For this review, take the finished solid that the model builds, in its own axes (mm). Coordinates: 2 decimals unless noted, no trailing zeros. Write each loop counter-clockwise with the first axis right and the second up, starting at its lowest first coordinate (ties: lowest second). Pieces come first, ordered by that corner, then holes.
1) To check wall thickness, follow line 1 along Y through (x, z) = (-34, 2.15); line 2 along Y through (x, z) = (-18.5, 2.45) (3 decimals); line 3 along X through (y, z) = (-4, 2.6). State the ranges of each line that lie inside material, in increasing order.
2) We need section C-C on x = -36.5. Write out the cut boundary in (y, z), then the cut area to 4 significant figures.
3) We need section A-A on z = 0.45. Write out the cut boundary in (x, y), then the cut area to 3 significant figures.
4) We need section B-B on y = -2. Write out the cut boundary in (x, z).
from build123d import *

# Parameters (mm, degrees)
F2_DEPTH    = 3
F3_T1_DEPTH = 3.3473896723


# Not quite as in the source:
# - a fillet or chamfer that OpenCascade refuses, or shapes differently, is made with other operations: its cross-section is extruded or revolved along the edge and cut away or added


with BuildPart() as f2:
    # F1 (on face) → F2 (new body)
    with BuildSketch(Plane.XY):
        with BuildLine():
            Line((23.5, -3.5), (20.4928553643, -3.3120534603))
            ThreePointArc((20.4928553643, -3.3120534603), (22.5915627309, -4.3550902955), (23.5, -6.5154699331))
            Line((23.5, -6.5154699331), (23.5, -3.5))
        make_face()
        with BuildLine():
            Line((-32.5, 7.5), (-32.5, 0))
            Line((-32.5, 0), (20.2037399466, -3.2939837467))
            ThreePointArc((20.2037399466, -3.2939837467), (20.3484922252, -3.2999054879), (20.4928553643, -3.3120534603))
            Line((20.4928553643, -3.3120534603), (23.5, -3.5))
            Line((23.5, -3.5), (23.5, -6.5154699331))
            ThreePointArc((23.5, -6.5154699331), (23.5030092301, -6.6577349666), (23.5, -6.8))
            Line((23.5, -6.8), (32.5, -7.5))
            Line((32.5, -7.5), (32.5, 7.5))
            Line((32.5, 7.5), (-32.5, 7.5))
        make_face()
        Polygon((-45, 0.78125), (-32.5, 0), (-32.5, 7.5), (-45, 7.5), align=None)
    extrude(amount=F2_DEPTH)

    # F3: fillet of radius 4 on 1 edges, made by hand

    # F3_s2 → F3_t1 (cut)
    with BuildSketch(Plane.XY.offset(-0.1736948361)):
        with BuildLine():
            ThreePointArc((20.134397315, -3.2896498322), (20.1925204005, -3.2928581253), (20.2506840199, -3.2952202421))
            ThreePointArc((20.2506840199, -3.2952202421), (20.2272141407, -3.2945200871), (20.2037399466, -3.2939837467))
            Line((20.2037399466, -3.2939837467), (20.134397315, -3.2896498322))
        make_face()
    extrude(amount=F3_T1_DEPTH, mode=Mode.SUBTRACT)


solid = f2.part
Result:
1. line 1: y = 0.09 to 7.5
1. line 2: y = -0.875 to 7.5
1. line 3: x = 22.2 to 32.5
2. outline: (0.25, 0) - (7.5, 0) - (7.5, 3) - (0.25, 3) - close
2. area: 21.75 mm2
3. outline: (-45, 0.78) - (20.13, -3.29) arc R4 ccw to (20.25, -3.3) arc R3.36 cw to (23.5, -6.8) - (32.5, -7.5) - (32.5, 7.5) - (-45, 7.5) - close
3. area: 741 mm2
4. outline: (-0.5, 0) - (32.5, 0) - (32.5, 3) - (-0.5, 3) - close
